from build123d import *

# Parameters (mm, degrees)
SKETCH_1_W          = 100
SKETCH_1_H          = 100
EXTRUDE_1_DEPTH     = 6
SKETCH_2_W          = 7
SKETCH_2_H          = 6
EXTRUDE_2_DEPTH     = 6
CUT_EXTRUDE_1_DEPTH = 7


with BuildPart() as part:
    # Эскиз1 → Бобышка-Вытянуть1 (new body)
    with BuildSketch(Plane.XY):
        Rectangle(SKETCH_1_W, SKETCH_1_H)
    extrude(amount=EXTRUDE_1_DEPTH)

    # Эскиз2 → Бобышка-Вытянуть2 (add)
    with BuildSketch(Plane.XY.offset(6)):
        with Locations((-9.531849908, 53)):
            Rectangle(SKETCH_2_W, SKETCH_2_H)
        with Locations((9.531849908, 53)):
            Rectangle(SKETCH_2_W, SKETCH_2_H)
    extrude(amount=-EXTRUDE_2_DEPTH)

    # Эскиз3 → Вырез-Вытянуть1 (cut, through all)
    with BuildSketch(Plane.XY.offset(6)):
        Polygon((-2.1, 42), (-3.6, 42), (-3.6, 39.6), (-2.1, 39.6), (-2.1, 35), (2.1, 35), (2.1, 39.6), (3.6, 39.6), (3.6, 42), (2.1, 42), (2.1, 50), (-2.1, 50), align=None)
    extrude(amount=-CUT_EXTRUDE_1_DEPTH, mode=Mode.SUBTRACT)


solid = part.part
Part model, mm, in its own coordinate system. A direction names the side the tool comes from. Coordinates: 2 decimals unless noted, no trailing zeros. Loops run counter-clockwise (first coordinate to the right, second up) from the corner with the lowest first, then second, coordinate; pieces in that order, holes last. Notation, with made-up numbers: (13.5, 7) -> (50.5, 7) arc R36 ccw to (50.5, 46) -> close; hole circle Ø3 at (87, 66). An arc over 180 degrees is marked (long way). Use a Markdown table: item, result. Add a question column.
Item 1: Which spindle directions (+Z, -Z, +X, -X, +Y, -Y) get a long thin tool onto all of the face, cutting with end or side? Do faces 4 (the flat face through (-3.6, 41, 3)), 5 (the flat face through (31, 50, 3)), 6 (the flat face through (-2.1, 46, 3)). Say none if no direction does.
Item 2: Band-saw the part on B-B on x = 23. Write the cut outline in (y, z), plus the area to 3 significant figures.
Item 3: Flat gauge pins, fed straight in: P1, Ø1.8, axis at x = -34.5, z = 2, coming from the +Y side; P2, Ø1.8, axis at y = 52, z = 4.5, coming from the +X side; P3, Ø3, axis at y = 52, z = 3.5, coming from the -X side. Where does each tip first touch, or does it go through?
Item 4: Band-saw the part on A-A on z = 4.65. Write the cut outline in (x, y).
Item 5: Probe probe 1 along X at (y, z) = (40.5, 4.55); probe 2 along Y at (x, z) = (-2.5, 5.2); probe 3 along Y at (x, z) = (30, 3.95). List the from-to ranges inside material, lowest first.
Item 6: Pull direction X, two halves, no side cores. Call faces 1 (the flat face through (-1, 4, 6)), 2 (the flat face through (-13.032, 53, 3)), 3 (the flat face through (-6.032, 53, 3)): +X half, -X half, draft (parallel to the pull), parting line (faces both ways), or undercut.
Geometry says:
| question | item | result |
|---|---|---|
| 1 | face 4 | +Z, -Z |
| 1 | face 5 | +Z, -Z, +X, +Y |
| 1 | face 6 | +Z, -Z, +Y |
| 2 | outline | (-50, 0) -> (50, 0) -> (50, 6) -> (-50, 6) -> close |
| 2 | area | 600 mm² |
| 3 | P1 | y = 50 |
| 3 | P2 | x = 13.03 |
| 3 | P3 | x = -13.03 |
| 4 | outline | (-50, -50) -> (50, -50) -> (50, 50) -> (13.03, 50) -> (13.03, 56) -> (6.03, 56) -> (6.03, 50) -> (2.1, 50) -> (2.1, 42) -> (3.6, 42) -> (3.6, 39.6) -> (2.1, 39.6) -> (2.1, 35) -> (-2.1, 35) -> (-2.1, 39.6) -> (-3.6, 39.6) -> (-3.6, 42) -> (-2.1, 42) -> (-2.1, 50) -> (-6.03, 50) -> (-6.03, 56) -> (-13.03, 56) -> (-13.03, 50) -> (-50, 50) -> close |
| 5 | probe 1 | -50 to -3.6, 3.6 to 50 |
| 5 | probe 2 | -50 to 39.6, 42 to 50 |
| 5 | probe 3 | -50 to 50 |
| 6 | face 1 | draft |
| 6 | face 2 | -X half |
| 6 | face 3 | undercut |
